Here's the drawing with two shaded views (mm, measured from the low corner). I have some questions. A direction names the side the tool comes from. Round coordinates to 2 decimals unless told otherwise and drop trailing zeros. Loops run counter-clockwise (first coordinate to the right, second up) from the corner with the lowest first, then second, coordinate; pieces in that order, holes last.
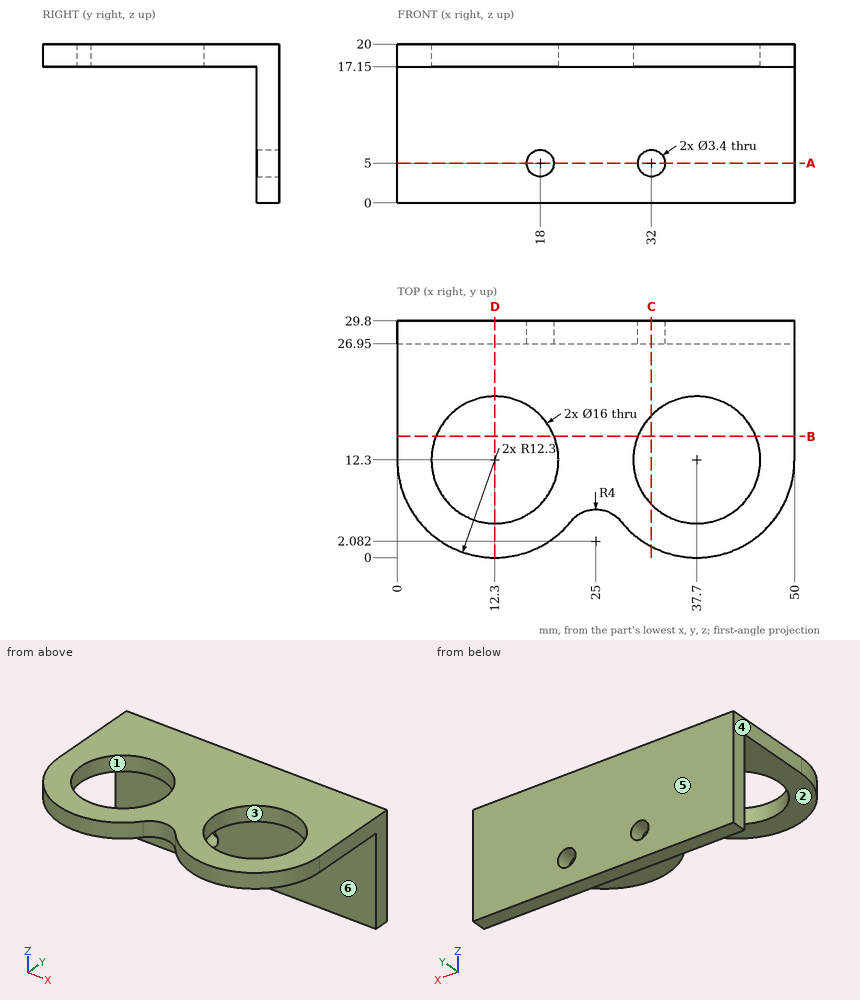
(1) If we section it at D-D, the plane x = 12.3: List the corners of the cut face in (y, z) for me.
Worked answers:
outline: (0, 17.15) - (4.3, 17.15) - (4.3, 20) - (0, 20) - close; (20.3, 17.15) - (26.95, 17.15) - (26.95, 0) - (29.8, 0) - (29.8, 20) - (20.3, 20) - close
(2) If we section it at A-A, the plane z = 5: List the corners of the cut face in (x, y) for me, then the cut area to 3 significant figures.
Worked answers:
outline: (0, 26.95) - (16.3, 26.95) - (16.3, 29.8) - (0, 29.8) - close; (19.7, 26.95) - (30.3, 26.95) - (30.3, 29.8) - (19.7, 29.8) - close; (33.7, 26.95) - (50, 26.95) - (50, 29.8) - (33.7, 29.8) - close
area: 123 mm2
(3) Will these pins go through, and if not, where does the flat tip stop? P1, Ø10, axis at y = 18, z = 13.5, coming from the -X side; P2, Ø10, axis at x = 41, z = 13, coming from the -Y side; P3, Ø8, axis at x = 30.5, y = 12, coming from the -Z side; P4, Ø5.5, axis at x = 18, z = 5, coming from the -Y side.
Worked answers:
P1: stops at x = 0
P2: stops at y = 0.01
P3: stops at z = 17.15
P4: stops at y = 26.95
(4) If I drill on line 1 (Y direction, x = 37.7, z = 18.45); line 2 (Z direction, x = 18, y = 27.9); line 3 (Y direction, x = 20, z = 6), over which ranges is the centre line in solid material (lowest first)?
Worked answers:
line 1: y = 0 to 4.3, 20.3 to 29.8
line 2: z = 0 to 3.3, 6.7 to 20
line 3: y = 26.95 to 29.8
(5) If we mould it in two halves opening along X, with no side actions, what happens to the marked faces 1, 2, 3 and 4? For each: released by +X, released by -X, zero draft, split by the parting line, or undercut.
Worked answers:
face 1: undercut
face 2: zero draft
face 3: undercut
face 4: released by -X
(6) If we section it at B-B, the plane y = 15.25: List the corners of the cut face in (x, z) for me.
Worked answers:
outline: (0, 17.15) - (4.86, 17.15) - (4.86, 20) - (0, 20) - close; (19.74, 17.15) - (30.26, 17.15) - (30.26, 20) - (19.74, 20) - close; (45.14, 17.15) - (50, 17.15) - (50, 20) - (45.14, 20) - close
(7) For the marked faces 5 and 6, which set-ups out of +Z, -Z, +X, -X, +Y, -Y let a thin tool reach every point of the face, with its end or its side?
Worked answers:
face 5: +Z, -Z, +X, -X, +Y
face 6: -Z, +X, -X, -Y
(8) If we section it at C-C, the plane x = 32: List the corners of the cut face in (y, z) for me.
Worked answers:
outline: (1.4, 17.15) - (6.69, 17.15) - (6.69, 20) - (1.4, 20) - close; (17.91, 17.15) - (26.95, 17.15) - (26.95, 6.7) - (29.8, 6.7) - (29.8, 20) - (17.91, 20) - close; (26.95, 0) - (29.8, 0) - (29.8, 3.3) - (26.95, 3.3) - close
